Geometry check sheet. Reference: the model listing, model coordinates, mm. A direction names the side the tool comes from. Give positions to 0.01 mm unless a question says otherwise; leave off trailing zeros. Order: outer loops, then holes, each group sorted by start corner. A loop starts at its lowest first (then second) coordinate and runs counter-clockwise, first axis right, second up. Notation, with made-up numbers: M 51,54 L 93,54 A26 ccw 93,71 Z; hole C -7,2.5 d8. An arc over 180 degrees is marked long. Answer as CSV lines item,"result".
from build123d import *

# Parameters (mm, degrees)
SKETCH1_W           = 35.5
SKETCH1_H           = 16.5
BOSS_EXTRUDE1_DEPTH = 1
SKETCH2_R           = 8.65
BOSS_EXTRUDE2_DEPTH = 18.6
SKETCH3_W           = 5
SKETCH3_H           = 8
BOSS_EXTRUDE3_DEPTH = 6.6


with BuildPart() as part:
    # Sketch1 → Boss-Extrude1 (new body)
    with BuildSketch(Plane(origin=(0, 0, 0), x_dir=(1, 0, 0), z_dir=(0, 1, 0))):
        Rectangle(SKETCH1_W, SKETCH1_H)
    extrude(amount=BOSS_EXTRUDE1_DEPTH)

    # Sketch2 → Boss-Extrude2 (add)
    with BuildSketch(Plane(origin=(0, 1, 0), x_dir=(1, 0, 0), z_dir=(0, 1, 0))):
        with Locations((-9.45, 0)):
            Circle(SKETCH2_R)
    extrude(amount=BOSS_EXTRUDE2_DEPTH)

    # Sketch3 → Boss-Extrude3 (add)
    with BuildSketch(Plane(origin=(0, 1, 0), x_dir=(1, 0, 0), z_dir=(0, 1, 0))):
        with Locations((11.337780318, -0.323708933)):
            Rectangle(SKETCH3_W, SKETCH3_H)
    extrude(amount=BOSS_EXTRUDE3_DEPTH)


solid = part.part
(1) Section check D-D on y = 9. Enter the section's corners in (x, z), then the cut area to 3 significant figures.
The answers:
outline,"C -9.45,0 d17.3"
area,"235 mm2"
(2) Section check B-B on y = 2. Enter the section's corners in (x, z), then the cut area to 3 significant figures.
The answers:
outline,"C -9.45,0 d17.3; M 8.84,-3.68 L 13.84,-3.68 L 13.84,4.32 L 8.84,4.32 Z"
area,"275 mm2"
(3) Gauge pin test, flat ends, axial feed: P1, Ø1.5, axis at x = 12, y = 6, coming from the -Z side; P2, Ø4, axis at x = 11, z = 1, coming from the +Y side; P3, Ø5, axis at y = 5, z = -3, coming from the -X side; P4, Ø8, axis at y = 2.5, z = -5.5, coming from the +X side. Record the tip position at first contact, or that the pin passes through.
The answers:
P1,"stops at z = -3.68"
P2,"stops at y = 7.6"
P3,"stops at x = -18.09"
P4,"stops at x = 17.75"
(4) Tool access check on faces 4 (the face through (11, 4, -3.676)), 5 (the face through (-18.09, 10.17, -0.38)), 6 (the face through (-16, 1, 6)), 7 (the face through (11, 7.6, 0)), 8 (the face through (11, 4, 4.324)). Record the directions out of +Z, -Z, +X, -X, +Y, -Y that give a thin tool (end or side, any length) a straight path to the whole face; none if there is none.
The answers:
face 4,"-Z, +X, +Y"
face 5,"+Y"
face 6,"+Z, -X, +Y"
face 7,"+Z, -Z, +X, +Y"
face 8,"+Z, +X, +Y"
(5) Draft check along X on faces 1 (the face through (8, 1, 0)), 2 (the face through (-17.75, 0.5, 0.1)), 3 (the face through (-16, 1, -7)). Enter one of: +X half, -X half, draft (parallel to the pull), parting line (faces both ways), or undercut.
The answers:
face 1,"undercut"
face 2,"-X half"
face 3,"draft"
(6) Section check A-A on z = 0. Enter the section's corners in (x, y), then the cut area to 3 significant figures.
The answers:
outline,"M -18.1,1 L -17.75,1 L -17.75,0 L 17.75,0 L 17.75,1 L 13.84,1 L 13.84,7.6 L 8.84,7.6 L 8.84,1 L -0.8,1 L -0.8,19.6 L -18.1,19.6 Z"
area,"390 mm2"
(7) Section check C-C on x = -4. Enter the section's corners in (y, z).
The answers:
outline,"M 0,-8.25 L 1,-8.25 L 1,-6.72 L 19.6,-6.72 L 19.6,6.72 L 1,6.72 L 1,8.25 L 0,8.25 Z"
(8) Material ranges on line 1 (Z direction, x = 9, y = 5.75); line 2 (Y direction, x = 0.5, z = -7); line 3 (Y direction, x = 9, z = 1), recorded low to high.
The answers:
line 1,"z = -3.68 to 4.32"
line 2,"y = 0 to 1"
line 3,"y = 0 to 7.6"
